Design review of the part built by this model. Coordinates are the model's own, in mm. A direction names the side the tool comes from. Coordinates: 2 decimals unless noted, no trailing zeros. Loops run counter-clockwise (first coordinate to the right, second up) from the corner with the lowest first, then second, coordinate; pieces in that order, holes last.
Q1. Draft analysis for pull direction X (two halves, no side actions). For faces 4 (the face through (-56.546, -10, 8)), 5 (the face through (-35, -13, 0)), 6 (the face through (44.25, -4.12, -2.76)), 7 (the face through (50.425, -4, 0)), state which applies: released by +X, released by -X, zero draft, split by the parting line, or undercut.
Q2. Add section A-A on z = -1. Give the boundary of the cut face in (x, y).
Q3. Add section D-D on y = -24.5. Give the boundary of the cut face in (x, z), and give its area (3 significant figures).
Q4. Add section C-C on x = -25. Give the boundary of the cut face in (y, z).
Q5. Wall thickness on probe 1 along X at (y, z) = (-18.75, 10); probe 2 along Y at (x, z) = (-9, 23); probe 3 along Z at (x, y) = (-16, -5): over which ranges is each line inside the solid? List them lowest first.
Q6. Add section B-B on x = 43. Give the boundary of the cut face in (y, z).
Q7. Machinability: for faces 1 (the face through (-51, -11, 27.253)), 2 (the face through (-26.111, -17.394, -6.107)), 3 (the face through (-45.47, -15, 10)), which of the approach directions +Z, -Z, +X, -X, +Y, -Y give a long, thin tool a straight path to every point of the face, cutting with its end or side? Answer none if there is none.
Q8. For P1, Ø16.5, axis at x = 37.6, z = 0, coming from the -Y side; P2, Ø8, axis at x = -39.5, y = -23, coming from the +Z side; P3, Ø2, axis at x = -50.5, y = -12, coming from the +Z side, all flat-tipped, find the tip position at first contact; note any pin that passes through.
```python
from build123d import *

# Parameters (mm, degrees)
F0_W      = 106.971476227
F0_H      = 54.2144235224
F1_DEPTH  = 8.128
F3_DEPTH  = 25.4
F4_R      = 7.2003845792
F5_DEPTH  = 25.4
F7_DEPTH  = 18.796
F9_DEPTH  = 25.4
F11_DEPTH = 25.4


with BuildPart() as f1:
    # F0 (on Front) → F1 (new body)
    with BuildSketch(Plane.XZ):
        with Locations((-3.0604917556, 14.7195057943)):
            Rectangle(F0_W, F0_H)
    extrude(amount=F1_DEPTH)

    # F2 (on face) → F3 (cut)
    with BuildSketch(Plane.XZ.offset(8.128)):
        Polygon((50.4252463579, 41.8267175555), (-23.2532570529, 41.8267175555), (50.4252463579, 13.3497529124), align=None)
    extrude(amount=-F3_DEPTH, mode=Mode.SUBTRACT)

    # F4 (on face) → F5 (cut)
    with BuildSketch(Plane.XZ.offset(8.128)):
        with Locations((37.6003310084, 0)):
            Circle(F4_R)
    extrude(amount=-F5_DEPTH, mode=Mode.SUBTRACT)

    # F6 (on face) → F7 (join)
    with BuildSketch(Plane.XZ.offset(8.128)):
        Polygon((-45.4701632261, 27.2529497743), (-56.5462298691, 27.2529497743), (-56.5462298691, -11.8047548458), (-7.286884822, -12.3877059668), (-7.286884822, 0), (-45.4701632261, 0), align=None)
    extrude(amount=F7_DEPTH)

    # F8 (on face) → F9 (cut)
    with BuildSketch(Plane.XY):
        Polygon((-7.286884822, -8.128), (-45.4701632261, -26.924), (-7.286884822, -26.924), align=None)
    extrude(amount=-F9_DEPTH, mode=Mode.SUBTRACT)

    # F10 (on face) → F11 (cut)
    with BuildSketch(Plane.YZ.offset(-45.4701632261)):
        Polygon((-26.924, 27.2529497743), (-26.924, 0), (-14.8652466014, 27.2529497743), align=None)
    extrude(amount=-F11_DEPTH, mode=Mode.SUBTRACT)


solid = f1.part
```
Entries:
1. face 4: released by -X
1. face 5: zero draft
1. face 6: undercut
1. face 7: released by +X
2. outline: (-56.55, -26.92) - (-45.47, -26.92) - (-7.29, -8.13) - (30.47, -8.13) - (30.47, 0) - (-56.55, 0) - close; (44.73, -8.13) - (50.43, -8.13) - (50.43, 0) - (44.73, 0) - close
3. outline: (-56.55, -11.8) - (-40.55, -11.99) - (-40.55, 0) - (-45.47, 0) - (-45.47, 5.48) - (-56.55, 5.48) - close
3. area: 251 mm2
4. outline: (-16.85, -12.18) - (-8.13, -12.18) - (-8.13, -12.39) - (0, -12.39) - (0, 41.83) - (-8.13, 41.83) - (-8.13, 0) - (-16.85, 0) - close
5. probe 1: x = -56.55 to -45.47
5. probe 2: y = -8.13 to 0
5. probe 3: z = -12.39 to 39.02
6. outline: (-8.13, -12.39) - (0, -12.39) - (0, -4.76) - (-8.13, -4.76) - close; (-8.13, 4.76) - (0, 4.76) - (0, 16.22) - (-8.13, 16.22) - close
7. face 1: +Z, +X, -X, -Y
7. face 2: +Z, -Z, +X, -Y
7. face 3: +Z, +X, -Y
8. P1: stops at y = -8.13
8. P2: stops at z = 0
8. P3: stops at z = 27.25
